from build123d import *

# Parameters (mm, degrees)
CYLINDER001_R     = 2.5
CYLINDER001_DEPTH = 7
FILLET_1_R        = 5
FILLET_2_R        = 0.9
FILLET_3_R        = 0.5
CYLINDER_R        = 9
CYLINDER_DEPTH    = 1
PAD_DEPTH         = 20
PAD001_DEPTH      = 20


with BuildPart() as handle_pocket:
    # Cylinder001 → Cylinder001 (new body)
    with BuildSketch(Plane.XY):
        Circle(CYLINDER001_R)
    extrude(amount=CYLINDER001_DEPTH)


with BuildPart() as base_fillet:
    # Sketch → Revolution (revolve)
    with BuildSketch(Plane.XZ):
        Polygon((0, 0), (4, 0), (4, 7), (8, 7), (10, 7.5), (10, 9), (9, 9), (9, 8), (0, 8), align=None)
    revolve(axis=Axis((0, 0, 0), (0, 0, 1)))

    # Fillet 1
    fillet_1_edges = [base_fillet.edges().sort_by_distance(p)[0] for p in [
        (-8, 0, 7),
    ]]
    fillet(fillet_1_edges, radius=FILLET_1_R)

    # Fillet 2
    fillet_2_edges = [base_fillet.edges().sort_by_distance(p)[0] for p in [
        (-10, 0, 9),
    ]]
    fillet(fillet_2_edges, radius=FILLET_2_R)

    # Fillet 3
    fillet_3_edges = [base_fillet.edges().sort_by_distance(p)[0] for p in [
        (-10, 0, 7.5),
    ]]
    fillet(fillet_3_edges, radius=FILLET_3_R)


with BuildPart() as obj1:
    # Cylinder → Cylinder (new body)
    with BuildSketch(Plane.XY.offset(4)):
        Circle(CYLINDER_R)
    extrude(amount=CYLINDER_DEPTH)


with BuildPart() as obj2:
    # MirroredSketch → Pad (new body)
    with BuildSketch(Plane.XZ.offset(-10)):
        Polygon((7.142857, 6.5), (5.714286, 4.5), (4.285714, 6.5), (2.857143, 4.5), (1.428571, 6.5), (0, 4.5), (-1.428571, 6.5), (-2.857143, 4.5), (-4.285714, 6.5), (-5.714286, 4.5), (-7.142857, 6.5), (-8.571429, 4.5), (-10, 6.5), (-10, 7.5), (10, 7.5), (10, 6.5), (8.571429, 4.5), align=None)
    extrude(amount=PAD_DEPTH)


with BuildPart() as handle:
    # MirroredSketch002 → Pad001 (new body)
    with BuildSketch(Plane.YZ.offset(-10)):
        Polygon((7.142857, 4.5), (5.714286, 6.5), (4.285714, 4.5), (2.857143, 6.5), (1.428571, 4.5), (0, 6.5), (-1.428571, 4.5), (-2.857143, 6.5), (-4.285714, 4.5), (-5.714286, 6.5), (-7.142857, 4.5), (-8.571429, 6.5), (-10, 4.5), (-10, 3.5), (10, 3.5), (10, 4.5), (8.571429, 6.5), align=None)
    extrude(amount=PAD001_DEPTH)

    # Cut: cut obj2
    add(obj2.part, mode=Mode.SUBTRACT)

    # Common: intersect obj1
    add(obj1.part, mode=Mode.INTERSECT)


with BuildPart() as handle_1:
    # Common placement: moved
    add(handle.part.moved(Location((0, 0, 4))))

    # Fusion: union Base Fillet
    add(base_fillet.part)

    # Cut001: cut Handle Pocket
    add(handle_pocket.part, mode=Mode.SUBTRACT)


solid = handle_1.part
Design review of the part built by this model. Coordinates are the model's own, in mm. Coordinates: 2 decimals unless noted, no trailing zeros. Order: outer loops, then holes, each group sorted by start corner. A loop starts at its lowest first (then second) coordinate and runs counter-clockwise, first axis right, second up.
Item 1: The part is to be moulded in two halves that separate along X. For faces 1 (the cylindrical face through (-0.867, -3.905, 3.549)), 2 (the flat face through (-1, -3, 9)), 3 (the flat face through (0, 0, 7)), say which applies: pulls with the +X half, pulls with the -X half, needs draft (parallel to the pull), parting line crosses it, or undercut.
Item 2: For pin 1 Ø4 at (y, z) = (-5, 1.5) entering from +X; pin 2 Ø5 at (x, z) = (-6, 7) entering from -Y; pin 3 Ø6 at (x, y) = (-7.5, -5) entering from -Z, all flat-tipped, find the tip position at first contact; note any pin that passes through.
Item 3: Take a section at A-A, the plane z = 6.25. Write out the cut boundary in (x, y), then the cut area to 3 significant figures.
Item 4: For line 1 (Y direction, x = 0, z = 3); line 2 (Z direction, x = -2.75, y = 2.5); line 3 (Z direction, x = 0.5, y = -6.25), list the stretches that pass through material, from the lowest coordinate up.
The answers:
1. face 1: parting line crosses it
1. face 2: needs draft
1. face 3: undercut
2. pin 1: stops at x = 2.65
2. pin 2: stops at y = -9.31
2. pin 3: stops at z = 7
3. outline: circle Ø8 at (0, 0); hole circle Ø5 at (0, 0)
3. area: 30.6 mm2
4. line 1: y = -4 to -2.5, 2.5 to 4
4. line 2: z = 0 to 8.65
4. line 3: z = 7 to 9
